```python
from build123d import *

# Parameters (mm, degrees)
SKETCH1_W           = 350
SKETCH1_H           = 250
BOSS_EXTRUDE1_DEPTH = 2
SKETCH2_OUTSIDE_W   = 438.024
SKETCH2_OUTSIDE_H   = 338.024
SKETCH2_OUTSIDE_R   = 1
CUT_EXTRUDE1_DEPTH  = 10


with BuildPart() as part:
    # Sketch1 → Boss-Extrude1 (new body)
    with BuildSketch(Plane(origin=(0, 0, 0), x_dir=(1, 0, 0), z_dir=(0, 1, 0))):
        with Locations((175, 125)):
            Rectangle(SKETCH1_W, SKETCH1_H)
    extrude(amount=BOSS_EXTRUDE1_DEPTH)

    # Sketch2 outside → Cut-Extrude1 (cut)
    with BuildSketch(Plane(origin=(0, 2, 0), x_dir=(1, 0, 0), z_dir=(0, 1, 0))):
        with Locations((175, 125)):
            Rectangle(SKETCH2_OUTSIDE_W, SKETCH2_OUTSIDE_H)
        with BuildLine():
            Line((20.622413462, 39.237304679), (20.622413462, 169.436764679))
            ThreePointArc((20.622413462, 169.436764679), (22.672665993, 174.386512147), (27.622413462, 176.436764679))
            Line((27.622413462, 176.436764679), (315.321763462, 176.436764679))
            ThreePointArc((315.321763462, 176.436764679), (320.27151093, 174.386512147), (322.321763462, 169.436764679))
            Line((322.321763462, 169.436764679), (322.321763462, 39.237304679))
            ThreePointArc((322.321763462, 39.237304679), (320.27151093, 34.28755721), (315.321763462, 32.237304679))
            Line((315.321763462, 32.237304679), (27.622413462, 32.237304679))
            ThreePointArc((27.622413462, 32.237304679), (22.672665993, 34.28755721), (20.622413462, 39.237304679))
        make_face(mode=Mode.SUBTRACT)
        with Locations((42.122413462, 172.436764679)):
            Circle(SKETCH2_OUTSIDE_R)
        with Locations((128.122413462, 172.436764679)):
            Circle(SKETCH2_OUTSIDE_R)
        with Locations((214.122413462, 172.436764679)):
            Circle(SKETCH2_OUTSIDE_R)
        with Locations((300.122413462, 172.686764679)):
            Circle(SKETCH2_OUTSIDE_R)
        with Locations((300.122413462, 36.237304679)):
            Circle(SKETCH2_OUTSIDE_R)
        with Locations((214.122413462, 35.987304679)):
            Circle(SKETCH2_OUTSIDE_R)
        with Locations((128.122413462, 35.987304679)):
            Circle(SKETCH2_OUTSIDE_R)
        with Locations((42.122413462, 35.987304679)):
            Circle(SKETCH2_OUTSIDE_R)
        with BuildLine():
            Line((312.821763462, 39.737304679), (30.122413462, 39.737304679))
            ThreePointArc((30.122413462, 39.737304679), (28.708199899, 40.323091116), (28.122413462, 41.737304679))
            Line((28.122413462, 41.737304679), (28.122413462, 134.737304679))
            ThreePointArc((28.122413462, 134.737304679), (28.708199899, 136.151518241), (30.122413462, 136.737304679))
            Line((30.122413462, 136.737304679), (312.821763462, 136.737304679))
            ThreePointArc((312.821763462, 136.737304679), (314.235977024, 136.151518241), (314.821763462, 134.737304679))
            Line((314.821763462, 134.737304679), (314.821763462, 41.737304679))
            ThreePointArc((314.821763462, 41.737304679), (314.235977024, 40.323091116), (312.821763462, 39.737304679))
        make_face()
    extrude(amount=-CUT_EXTRUDE1_DEPTH, mode=Mode.SUBTRACT)


solid = part.part
```
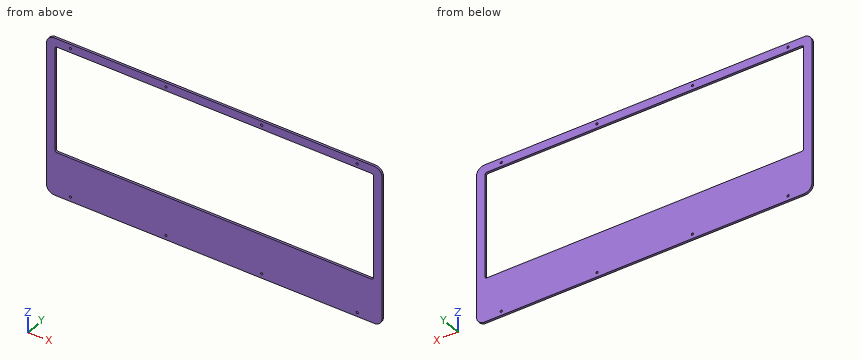
The model under review builds one solid part; all positions refer to its coordinate system, in mm. Round coordinates to 2 decimals unless told otherwise and drop trailing zeros. Loops run counter-clockwise (first coordinate to the right, second up) from the corner with the lowest first, then second, coordinate; pieces in that order, holes last. Notation, with made-up numbers: M 49.5,60 L 96.5,60 A27 cw 96.5,86 Z; hole C 32,-25 d1. An arc over 180 degrees is marked long. Answer as a JSON object with one key per item and string values.
(1) Take a section at A-A on x = 136. Give the boundary of the cut face in (y, z).
Resolved:
{"outline": "M 0,-176.44 L 2,-176.44 L 2,-136.74 L 0,-136.74 Z; M 0,-39.74 L 2,-39.74 L 2,-32.24 L 0,-32.24 Z"}
(2) Clearance check with a flat-ended pin moving along its axis: P1, Ø1.2, axis at x = 42.12, z = -172.44, coming from the -Y side. State where the tip first meets the part, or that it passes through.
Resolved:
{"P1": "through"}
(3) Take a section at B-B on z = -114. Give the boundary of the cut face in (x, y), and give its area (3 significant figures).
Resolved:
{"outline": "M 20.62,0 L 28.12,0 L 28.12,2 L 20.62,2 Z; M 314.82,0 L 322.32,0 L 322.32,2 L 314.82,2 Z", "area": "30.0 mm²"}
(4) To check wall thickness, follow line 1 along Z through (x, y) = (65, 1.35); line 2 along X through (y, z) = (1.25, -114); line 3 along X through (y, z) = (1.3, -136.5). State the ranges of each line that lie inside material, in increasing order.
Resolved:
{"line 1": "-176.44 to -136.74, -39.74 to -32.24", "line 2": "20.62 to 28.12, 314.82 to 322.32", "line 3": "20.62 to 29.18, 313.77 to 322.32"}
(5) Take a section at C-C on y = 0.35. Count the separate pieces of the cut face and the enclosed holes in it, and give its area (3 significant figures).
Resolved:
{"separate pieces": "1", "enclosed holes": "9", "area": "15,600 mm²"}
